Verification items for the finished model (mm, model axes). A direction names the side the tool comes from. Coordinates: 2 decimals unless noted, no trailing zeros. Loops run counter-clockwise (first coordinate to the right, second up) from the corner with the lowest first, then second, coordinate; pieces in that order, holes last.
Q1. Material ranges on probe 1 along X at (y, z) = (18.25, 30); probe 2 along X at (y, z) = (-0.65, 0); probe 3 along Z at (x, y) = (-34, 8.5), recorded low to high.
Q2. Go/stop test with a flat-tipped pin: P1, Ø12, axis at x = 30, z = -30, coming from the -Y side. Record where the tip stops, or that it passes through.
Q3. Mould release check, pull along X, two halves, no side actions. Record for faces 1 (the face through (-19, -3, 7)), 2 (the face through (33.55, 12.32, -33.87)), 3 (the face through (44, 12, 0)): +X half, -X half, draft (parallel to the pull), parting line (faces both ways), or undercut.
Q4. Access from +Z, -Z, +X, -X, +Y, -Y to the whole of each face (thin tool, end or side, straight path). Record for faces 4 (the face through (-15.88, -1.48, -17.32)), 5 (the face through (7.21, 23.52, 22.89)), 6 (the face through (-40, 12.3, 39.8)).
Q5. Sectioned sample at B-B (x = 0). Enter the section's corners in (y, z).
Q6. Sectioned sample at D-D (x = -34). Enter the section's corners in (y, z).
Q7. Sectioned sample at C-C (y = 15.75). Enter the section's corners in (x, z), then the cut area to 3 significant figures.
Q8. Sectioned sample at A-A (z = 0). Enter the section's corners in (x, y), then the cut area to 3 significant figures.
```python
from build123d import *

# Parameters (mm, degrees)
ESQUISSE1_R             = 5.25
ESQUISSE1_R_2           = 20
BOSS_EXTRU_1_DEPTH      = 25
ESQUISSE2_R             = 24
ENL_V_MAT_EXTRU_1_DEPTH = 3
ESQUISSE3_R             = 23.5
ESQUISSE3_R_2           = 20
BOSS_EXTRU_2_DEPTH      = 3


with BuildPart() as part:
    # Esquisse1 → Boss.-Extru.1 (new body)
    with BuildSketch(Plane(origin=(0, 0, 0), x_dir=(1, 0, 0), z_dir=(0, 1, 0))):
        with BuildLine():
            Line((-44, 30), (-44, -30))
            ThreePointArc((-44, -30), (-39.899495706, -39.899494167), (-30.000002176, -44))
            Line((-30.000002176, -44), (30, -44))
            ThreePointArc((30, -44), (39.899494937, -39.899494937), (44, -30))
            Line((44, -30), (44, 30))
            ThreePointArc((44, 30), (39.899494937, 39.899494937), (30, 44))
            Line((30, 44), (-30.000002176, 44))
            ThreePointArc((-30.000002176, 44), (-39.899495706, 39.899494167), (-44, 30))
        make_face()
        with Locations(Location((-30, 30, 0), (0, 0, 270))):  # turned: the seam where the file's is
            Circle(ESQUISSE1_R, mode=Mode.SUBTRACT)
        with Locations(Location((30, 30, 0), (0, 0, 270))):  # turned: the seam where the file's is
            Circle(ESQUISSE1_R, mode=Mode.SUBTRACT)
        with Locations(Location((30, -30, 0), (0, 0, 270))):  # turned: the seam where the file's is
            Circle(ESQUISSE1_R, mode=Mode.SUBTRACT)
        with Locations(Location((-30, -30, 0), (0, 0, 270))):  # turned: the seam where the file's is
            Circle(ESQUISSE1_R, mode=Mode.SUBTRACT)
        with Locations(Location((0, 0, 0), (0, 0, 270))):  # turned: the seam where the file's is
            Circle(ESQUISSE1_R_2, mode=Mode.SUBTRACT)
    extrude(amount=BOSS_EXTRU_1_DEPTH)

    # Esquisse2 → Enlèv. mat.-Extru.1 (cut)
    with BuildSketch(Plane(origin=(0, 25, 0), x_dir=(1, 0, 0), z_dir=(0, 1, 0))):
        with Locations(Location((0, 0, 0), (0, 0, 270))):  # turned: the seam where the file's is
            Circle(ESQUISSE2_R)
    extrude(amount=-ENL_V_MAT_EXTRU_1_DEPTH, mode=Mode.SUBTRACT)

    # Esquisse3 → Boss.-Extru.2 (add)
    with BuildSketch(Plane.XZ):
        with Locations(Location((0, 0, 0), (0, 0, 90))):  # turned: the seam where the file's is
            Circle(ESQUISSE3_R)
        with Locations(Location((0, 0, 0), (0, 0, 270))):  # turned: the seam where the file's is
            Circle(ESQUISSE3_R_2, mode=Mode.SUBTRACT)
    extrude(amount=BOSS_EXTRU_2_DEPTH)


solid = part.part
```
Geometry check:
1. probe 1: x = -44 to -35.25, -24.75 to 24.75, 35.25 to 44
1. probe 2: x = -23.5 to -20, 20 to 23.5
1. probe 3: z = -43.42 to -33.4, -26.6 to 26.6, 33.4 to 43.42
2. P1: stops at y = 0
3. face 1: draft
3. face 2: undercut
3. face 3: +X half
4. face 4: -Y
4. face 5: +Y
4. face 6: +Z, -X, +Y, -Y
5. outline: (-3, -23.5) - (0, -23.5) - (0, -44) - (25, -44) - (25, -24) - (22, -24) - (22, -20) - (-3, -20) - close; (-3, 20) - (22, 20) - (22, 24) - (25, 24) - (25, 44) - (0, 44) - (0, 23.5) - (-3, 23.5) - close
6. outline: (0, -43.42) - (25, -43.42) - (25, -33.4) - (0, -33.4) - close; (0, -26.6) - (25, -26.6) - (25, 26.6) - (0, 26.6) - close; (0, 33.4) - (25, 33.4) - (25, 43.42) - (0, 43.42) - close
7. outline: (-44, -30) arc R14 ccw to (-30, -44) - (30, -44) arc R14 ccw to (44, -30) - (44, 30) arc R14 ccw to (30, 44) - (-30, 44) arc R14 ccw to (-44, 30) - close; hole circle Ø10.5 at (-30, -30); hole circle Ø10.5 at (-30, 30); hole circle Ø40 at (0, 0); hole circle Ø10.5 at (30, -30); hole circle Ø10.5 at (30, 30)
7. area: 5,970 mm2
8. outline: (-44, 0) - (-23.5, 0) - (-23.5, -3) - (-20, -3) - (-20, 22) - (-24, 22) - (-24, 25) - (-44, 25) - close; (20, -3) - (23.5, -3) - (23.5, 0) - (44, 0) - (44, 25) - (24, 25) - (24, 22) - (20, 22) - close
8. area: 1,200 mm2
